Part model, mm, in its own coordinate system. A direction names the side the tool comes from. Coordinates: 2 decimals unless noted, no trailing zeros. Loops run counter-clockwise (first coordinate to the right, second up) from the corner with the lowest first, then second, coordinate; pieces in that order, holes last. Notation, with made-up numbers: (72, 75.5) -> (84, 75.5) arc R14 cw to (84, 100.5) -> close; hole circle Ø4 at (-23.75, 43). An arc over 180 degrees is marked (long way). Use one line per item in the form item = value. Start each with the question number.
(1) Mould opens along X. For faces 1 (the flat face through (144.801, 1.93, -843.04)), 2 (the cylindrical face through (145.37, 5.641, -844.086)), 3 (the flat face through (153, 9, -838.713)) say: +X half, -X half, draft (parallel to the pull), parting line (faces both ways), or undercut.
(2) Band-saw the part on D-D on z = -826.25. Give the cut face in (x, y) (3 decimals).
(3) Drill centre lines: L1, parallel to X at y = 11.25, z = -833.75; L2, parallel to Y at x = 149, z = -833.25; L3, parallel to Y at x = 180, z = -835 (3 decimals). Where is each one in solid material? Low to high. Write a range as [from, to].
(4) Pin check, flat tips, straight feed: P1, Ø1.4, axis at x = 154, y = 8, coming from the +Z side; P2, Ø3.5, axis at x = 152.5, y = -10, coming from the +Z side; P3, Ø2.5, axis at x = 153, y = -11, coming from the -Z side. Stop position of each tip, or through.
(5) 3-axis set-ups, long thin cutter, end or side, ignore diameter. For faces 4 (the flat face through (153, -9, -838.713)), 5 (the cylindrical face through (155.62, 7.728, -846.807)), 6 (the flat face through (179, -3.175, -837)), 7 (the flat face through (159.088, 0, -837)), 8 (the flat face through (179, 3.175, -837)): which of +Z, -Z, +X, -X, +Y, -Y reach the whole face in a straight line?
(6) Band-saw the part on A-A on y = -8.25. Give the cut face in (x, z), then the cut area to 3 significant figures.
(7) Band-saw the part on B-B on x = 174. Give the cut face in (y, z) (3 decimals), then the cut area to 3 significant figures.
```python
from build123d import *

# Parameters (mm, degrees)
CUT_EXTRUDE1_DEPTH      = 869.726648215
CUT_EXTRUDE1_DEPTH_BACK = 869.726648215
SKETCH2_3_R             = 8.334375
SKETCH3_R               = 6.44921875
CUT_EXTRUDE2_DEPTH      = 14.2875
CUT_EXTRUDE4_DEPTH      = 184.852841047


with BuildPart() as part:
    # Sketch2 one side → Revolve1 (revolve)
    with BuildSketch(Plane(origin=(0, 0, 0), x_dir=(1, 0, 0), z_dir=(0, 1, 0)), mode=Mode.PRIVATE) as revolve1_sk:
        with BuildLine():
            Line((161.802656837, 836.728797606), (178.471406837, 836.728797606))
            ThreePointArc((178.471406837, 836.728797606), (170.137031837, 845.063172606), (161.802656837, 836.728797606))
        make_face()
        with BuildLine():
            Line((155.119281837, 838.713172606), (150.479125, 838.713172606))
            ThreePointArc((150.479125, 838.713172606), (149.075959981, 838.131962625), (148.49475, 836.728797606))
            Line((148.49475, 836.728797606), (157.103656837, 836.728797606))
            ThreePointArc((157.103656837, 836.728797606), (156.522446856, 838.131962625), (155.119281837, 838.713172606))
        make_face()
        Polygon((144.800531837, 845.999797606), (144.800531837, 836.728797606), (181.646406837, 836.728797606), (181.646406837, 849.428797606), (145.956231837, 849.428797606), (145.956231837, 845.999797606), align=None)
    revolve(revolve1_sk.sketch.rotate(Axis((144.800531837, 0, -836.728797606), (1, 0, 0)), 180), axis=Axis((144.800531837, 0, -836.728797606), (1, 0, 0)))

    # Sketch2<3> → Cut-Extrude1 (cut, two sides: drawn at the far end of the back side and taken through both)
    with BuildSketch(Plane(origin=(0, 0, 0), x_dir=(1, 0, 0), z_dir=(0, 1, 0)).offset(-CUT_EXTRUDE1_DEPTH_BACK)):
        with Locations(Location((170.137031837, 836.728797606, 0), (0, 0, 270))):
            Circle(SKETCH2_3_R)
        with BuildLine():
            Line((150.479125, 838.713172606), (155.119281837, 838.713172606))
            ThreePointArc((155.119281837, 838.713172606), (157.103656837, 836.728797606), (155.119281837, 834.744422606))
            Line((155.119281837, 834.744422606), (150.479125, 834.744422606))
            ThreePointArc((150.479125, 834.744422606), (148.49475, 836.728797606), (150.479125, 838.713172606))
        make_face()
    extrude(amount=CUT_EXTRUDE1_DEPTH + CUT_EXTRUDE1_DEPTH_BACK, mode=Mode.SUBTRACT)

    # Sketch3 → Cut-Extrude2 (cut)
    with BuildSketch(Plane.ZY.offset(-144.800531837)):
        with Locations((-836.728797606, 0)):
            Circle(SKETCH3_R)
    extrude(amount=-CUT_EXTRUDE2_DEPTH, mode=Mode.SUBTRACT)

    # Sketch5 → Cut-Extrude4 (cut, through all)
    with BuildSketch(Plane.XY.offset(-824.028797606)):
        with BuildLine():
            Line((168.152656837, 3.175), (181.646406837, 3.175))
            Line((181.646406837, 3.175), (181.646406837, 12.7))
            Line((181.646406837, 12.7), (161.802656837, 12.7))
            Line((161.802656837, 12.7), (161.802656837, 9.525))
            ThreePointArc((161.802656837, 9.525), (163.662528777, 5.034871939), (168.152656837, 3.175))
        make_face()
        with BuildLine():
            Line((161.802656837, -12.7), (181.646406837, -12.7))
            Line((181.646406837, -12.7), (181.646406837, -3.175))
            Line((181.646406837, -3.175), (168.152656837, -3.175))
            ThreePointArc((168.152656837, -3.175), (163.662528777, -5.034871939), (161.802656837, -9.525))
            Line((161.802656837, -9.525), (161.802656837, -12.7))
        make_face()
    extrude(amount=-CUT_EXTRUDE4_DEPTH, mode=Mode.SUBTRACT)


solid = part.part
```
A:
q1.face_1 = -X half
q1.face_2 = draft
q1.face_3 = undercut
q2.outline = (145.956, -7.175) -> (162.253, -7.175) arc R6.35 cw to (168.153, -3.175) -> (181.646, -3.175) -> (181.646, 3.175) -> (168.153, 3.175) arc R6.35 cw to (162.253, 7.175) -> (145.956, 7.175) -> close
q3.L1 = [145.96, 161.8]
q3.L2 = [-12.21, -5.43], [5.43, 12.21]
q3.L3 = [-3.175, 3.175]
q4.P1 = -826.34
q4.P2 = -827.07
q4.P3 = -844.87
q5.face_4 = +Y, -Y
q5.face_5 = +X, -X
q5.face_6 = +Z, -Z, +X, -Y
q5.face_7 = -X
q5.face_8 = +Z, -Z, +X, +Y
q6.outline = (144.8, -840.96) -> (145.96, -840.96) -> (145.96, -846.38) -> (161.93, -846.38) -> (161.93, -838.19) arc R8.33 cw to (161.93, -835.27) -> (161.93, -827.07) -> (145.96, -827.07) -> (145.96, -832.5) -> (144.8, -832.5) -> close; hole (150.48, -838.71) -> (155.12, -838.71) arc R1.98 ccw to (155.12, -834.74) -> (150.48, -834.74) arc R1.98 ccw to start
q6.area = 287 mm²
q7.outline = (-3.175, -849.026) arc R12.7 ccw to (3.175, -849.026) -> (3.175, -844.114) -> (-3.175, -844.114) -> close; (-3.175, -829.344) -> (3.175, -829.344) -> (3.175, -824.432) arc R12.7 ccw to (-3.175, -824.432) -> close
q7.area = 65.8 mm²
